from build123d import *

# Parameters (mm, degrees)
F0_R     = 10
F1_DEPTH = 30
F3_D     = 16.5
F3_DEPTH = 20
F3_TIP   = 4.957100107
F5_D     = 8.2
F5_DEPTH = 100
F5_START = 22.4935716
F5_TIP   = 2.463528538


with BuildPart() as f1:
    # F0 (on Front) → F1 (new body)
    with BuildSketch(Plane.XZ):
        Circle(F0_R)
    extrude(amount=F1_DEPTH)

    # F3
    with Locations(Plane(origin=(0, 0, 0), x_dir=(1, 0, 0), z_dir=(0, 1, 0))):
        with Locations((0, 0)):
            Hole(F3_D / 2, depth=F3_DEPTH)
            with Locations((0, 0, -(F3_DEPTH + F3_TIP / 2))):  # 118° drill point
                Cone(0, F3_D / 2, F3_TIP, mode=Mode.SUBTRACT)

    # F5
    # its depths count from where the whole tool has entered the part; down to there all is cleared
    with Locations(Plane(origin=(0, 0, 0), x_dir=(1, 0, 0), z_dir=(0, 1, 0)).offset(-F5_START)):
        with Locations((0, 0)):
            Hole(F5_D / 2, depth=F5_DEPTH)
            with Locations((0, 0, -(F5_DEPTH + F5_TIP / 2))):  # 118° drill point
                Cone(0, F5_D / 2, F5_TIP, mode=Mode.SUBTRACT)


solid = f1.part
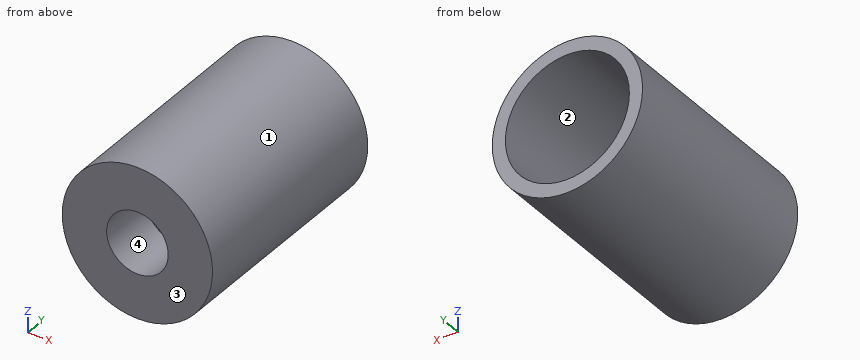
Could you check a few things on this model? Use its own coordinates, in mm. Face numbers are marked on the shaded views. Coordinates: 2 decimals unless noted, no trailing zeros. Write each loop counter-clockwise with the first axis right and the second up, starting at its lowest first coordinate (ties: lowest second). Pieces come first, ordered by that corner, then holes. Notation, with made-up numbers: M 54.25,56.5 L 89.25,56.5 A31 cw 89.25,85.5 Z; hole C 43,46 d3. An arc over 180 degrees is marked long. One line per question, with ' | ' between items.
1) Imagine slicing it at A-A, the plane z = 0. Write out the boundary of the cut face in (x, y).
Checks:
outline: M -10,-30 L -4.1,-30 L -4.1,-22.49 L -8.25,-20 L -8.25,0 L -10,0 Z; M 4.1,-30 L 10,-30 L 10,0 L 8.25,0 L 8.25,-20 L 4.1,-22.49 Z
2) Imagine slicing it at D-D, the plane y = -3.5. Write out the boundary of the cut face in (x, z), and give its area (3 significant figures).
Checks:
outline: C 0,0 d20; hole C 0,0 d16.5 | area: 100 mm²
3) I need wall thicknesses on probe 1 along Z at (x, y) = (0, -15.75); probe 2 along Z at (x, y) = (3.5, -24.5); probe 3 along X at (y, z) = (-11.25, -7.25). Which ranges of each line are inside material? Lowest first, please. Write a range as [from, to].
Checks:
probe 1: [-10, -8.25], [8.25, 10] | probe 2: [-9.37, -2.14], [2.14, 9.37] | probe 3: [-6.89, -3.94], [3.94, 6.89]
4) For pin 1 Ø3 at (x, y) = (-3, -22) entering from +Z; pin 2 Ø5 at (y, z) = (-15.5, -3) entering from -X; pin 3 Ø12 at (x, y) = (6.5, -13) entering from +Z; pin 4 Ø7.5 at (x, z) = (0, 0) entering from +Y, each with a flat end and sliding along its axis, tell me the tip position at first contact or that it passes through.
Checks:
pin 1: z = 9.89 | pin 2: x = -9.99 | pin 3: z = 9.99 | pin 4: through
5) Imagine slicing it at C-C, the plane y = -27.75. Write out the boundary of the cut face in (x, z), and give its area (3 significant figures).
Checks:
outline: C 0,0 d20; hole C 0,0 d8.2 | area: 261 mm²
6) If we mould it in two halves opening along X, with no side actions, what happens to the marked faces 1, 2, 3 and 4? For each: released by +X, released by -X, zero draft, split by the parting line, or undercut.
Checks:
face 1: split by the parting line | face 2: undercut | face 3: zero draft | face 4: undercut
7) Imagine slicing it at B-B, the plane x = 0. Write out the boundary of the cut face in (y, z).
Checks:
outline: M -30,-10 L 0,-10 L 0,-8.25 L -20,-8.25 L -22.49,-4.1 L -30,-4.1 Z; M -30,4.1 L -22.49,4.1 L -20,8.25 L 0,8.25 L 0,10 L -30,10 Z
